Design review of the part built by this model. Coordinates are the model's own, in mm. Face numbers are marked on the shaded views. Give positions to 0.01 mm unless a question says otherwise; leave off trailing zeros. Order: outer loops, then holes, each group sorted by start corner. A loop starts at its lowest first (then second) coordinate and runs counter-clockwise, first axis right, second up. Notation, with made-up numbers: (-1, 8) -> (35, 8) arc R11 ccw to (35, 13) -> close; hole circle Ø1 at (36.25, 10.25). An arc over 180 degrees is marked (long way). Return JSON: item names as keys, results as strings.
```python
from build123d import *

# Parameters (mm, degrees)
SKETCH_W     = 60
SKETCH_H     = 30
SKETCH_W_2   = 50
SKETCH_H_2   = 20
PAD_DEPTH    = 4
CHAMFER_SIZE = 2


with BuildPart() as part:
    # Sketch → Pad (new body)
    with BuildSketch(Plane.XY):
        Rectangle(SKETCH_W, SKETCH_H)
        Rectangle(SKETCH_W_2, SKETCH_H_2, mode=Mode.SUBTRACT)
    extrude(amount=PAD_DEPTH)

    # Chamfer
    chamfer_edges = [part.edges().sort_by_distance(p)[0] for p in [
        (0, -15, 4),
        (30, 0, 4),
        (0, 15, 4),
        (-30, 0, 4),
    ]]
    chamfer(chamfer_edges, length=CHAMFER_SIZE)


solid = part.part
```
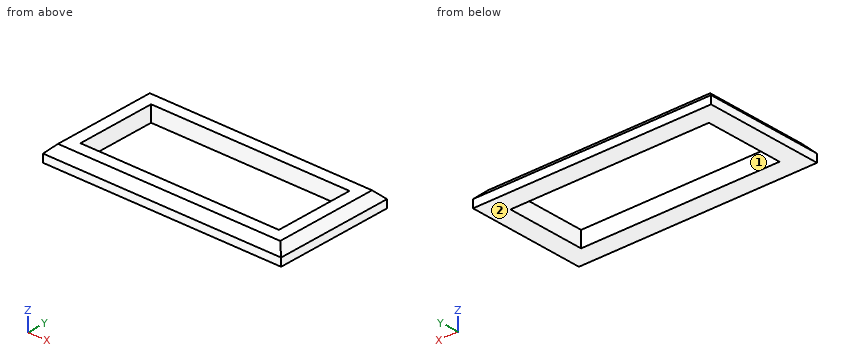
Item 1: Add section B-B (x = 10.5). Give the boundary of the cut face in (y, z), plus the area to 3 significant figures.
Result set:
{"outline": "(-15, 0) -> (-10, 0) -> (-10, 4) -> (-13, 4) -> (-15, 2) -> close; (10, 0) -> (15, 0) -> (15, 2) -> (13, 4) -> (10, 4) -> close", "area": "36.0 mm^2"}
Item 2: For pin 1 (2 mm diameter, centred on x = -7.5, z = 2.5, fed in from -Y); pin 2 (2 mm diameter, centred on x = 20.5, z = 3.5, fed in from -Y), all flat-tipped, find the tip position at first contact; note any pin that passes through.
Result set:
{"pin 1": "stops at y = -15", "pin 2": "stops at y = -14.5"}
Item 3: Mouldability with a two-part tool opening along Y and no side actions: class the marked faces 1 and 2 as released by +Y, released by -Y, zero draft, split by the parting line, or undercut.
Result set:
{"face 1": "undercut", "face 2": "zero draft"}
Item 4: Wall thickness on L1, parallel to X at y = -7, z = 1.3; L2, parallel to Y at x = 18, z = 0.85; L3, parallel to Y at x = -7.5, z = 2.9: over which ranges is each line inside the solid? List them lowest first. Write a range as [from, to].
Result set:
{"L1": "x = [-30, -25], [25, 30]", "L2": "y = [-15, -10], [10, 15]", "L3": "y = [-14.1, -10], [10, 14.1]"}
Item 5: Add section A-A (y = 4.5). Give the boundary of the cut face in (x, z), plus the area to 3 significant figures.
Result set:
{"outline": "(-30, 0) -> (-25, 0) -> (-25, 4) -> (-28, 4) -> (-30, 2) -> close; (25, 0) -> (30, 0) -> (30, 2) -> (28, 4) -> (25, 4) -> close", "area": "36.0 mm^2"}
Item 6: Add section C-C (z = 0.6). Give the boundary of the cut face in (x, y).
Result set:
{"outline": "(-30, -15) -> (30, -15) -> (30, 15) -> (-30, 15) -> close; hole (-25, -10) -> (25, -10) -> (25, 10) -> (-25, 10) -> close"}
